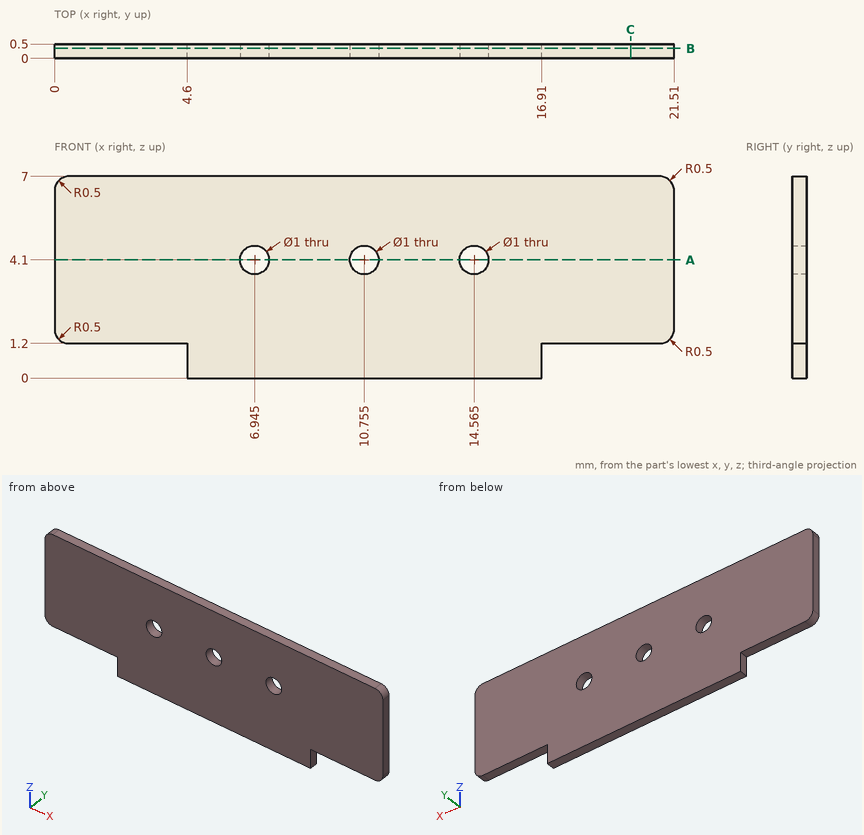
Design review of the part shown in the three views and the two pictorial views. Dimensions are in mm from the part's minimum x, y and z. Round coordinates to 2 decimals unless told otherwise and drop trailing zeros. Loops run counter-clockwise (first coordinate to the right, second up) from the corner with the lowest first, then second, coordinate; pieces in that order, holes last. Notation, with made-up numbers: (79, 5) -> (89, 5) arc R25 ccw to (89, 21) -> close; hole circle Ø7 at (47, -11.75). An arc over 180 degrees is marked (long way). Answer as a JSON object with one key per item and string values. Group by question number.
1) For line 1 (X direction, y = 0.1, z = 4.1) (3 decimals); line 2 (X direction, y = 0.25, z = 1); line 3 (Z direction, x = 15, y = 0.1), list the stretches that pass through material, from the lowest coordinate up. Write a range as [from, to].
2) For pin 1 Ø1.5 at (x, z) = (7, 4.5) entering from -Y, flat-tipped, find the tip position at first contact; note if it passes through.
3) We need section A-A on z = 4.1. Write out the cut boundary in (x, y) (3 decimals), then the cut area to 4 significant figures.
4) We need section C-C on x = 20. Write out the cut boundary in (y, z).
5) We need section B-B on y = 0.35. Write out the cut boundary in (x, z) (3 decimals), then the cut area to 3 significant figures.
Result set:
{
 "1": {"line 1": "[0, 6.445], [7.445, 10.255], [11.255, 14.065], [15.065, 21.51]", "line 2": "[4.6, 16.91]", "line 3": "[0, 3.85], [4.35, 7]"},
 "2": {"pin 1": "y = 0"},
 "3": {"outline": "(0, 0) -> (6.445, 0) -> (6.445, 0.5) -> (0, 0.5) -> close; (7.445, 0) -> (10.255, 0) -> (10.255, 0.5) -> (7.445, 0.5) -> close; (11.255, 0) -> (14.065, 0) -> (14.065, 0.5) -> (11.255, 0.5) -> close; (15.065, 0) -> (21.51, 0) -> (21.51, 0.5) -> (15.065, 0.5) -> close", "area": "9.255 mm²"},
 "4": {"outline": "(0, 1.2) -> (0.5, 1.2) -> (0.5, 7) -> (0, 7) -> close"},
 "5": {"outline": "(0, 1.7) arc R0.5 ccw to (0.5, 1.2) -> (4.6, 1.2) -> (4.6, 0) -> (16.91, 0) -> (16.91, 1.2) -> (21.01, 1.2) arc R0.5 ccw to (21.51, 1.7) -> (21.51, 6.5) arc R0.5 ccw to (21.01, 7) -> (0.5, 7) arc R0.5 ccw to (0, 6.5) -> close; hole circle Ø1 at (6.945, 4.1); hole circle Ø1 at (10.755, 4.1); hole circle Ø1 at (14.565, 4.1)", "area": "137 mm²"}
}
